Here's how the part is built. I have some questions about the finished solid (model axes, mm). Round coordinates to 2 decimals unless told otherwise and drop trailing zeros. Order: outer loops, then holes, each group sorted by start corner. A loop starts at its lowest first (then second) coordinate and runs counter-clockwise, first axis right, second up.
```python
from build123d import *

# Parameters (mm, degrees)
VACIADO2_T            = -2
CROQUIS2_R            = 3
CORTAR_EXTRUIR1_DEPTH = 26.980762114


with BuildPart() as part:
    # Croquis1 → Revolución1 (revolve)
    with BuildSketch(Plane.XY):
        with BuildLine():
            Line((0, 0), (0, 15))
            ThreePointArc((0, 15), (-10.606601718, 10.606601718), (-15, 0))
            Line((-15, 0), (0, 0))
        make_face()
    revolve(axis=Axis((0, 0, 0), (0, 1, 0)))

    # Vaciado2
    vaciado2_openings = [part.faces().sort_by_distance(p)[0] for p in [
        (0, 0, 0),
    ]]
    offset(amount=VACIADO2_T, openings=vaciado2_openings, kind=Kind.INTERSECTION)

    # Croquis2 → Cortar-Extruir1 (cut, through all)
    with BuildSketch(Plane.XY):
        with Locations(Location((0, 8.456456299, 0), (0, 0, 111.940512479))):
            Circle(CROQUIS2_R)
    extrude(amount=CORTAR_EXTRUIR1_DEPTH, mode=Mode.SUBTRACT)


solid = part.part
```
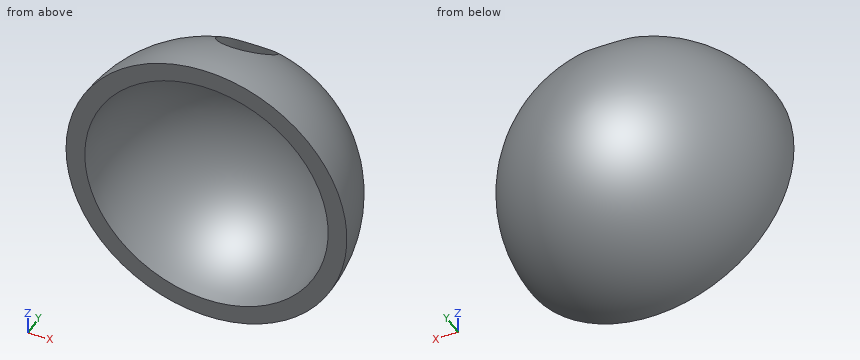
1. I need wall thicknesses on probe 1 along X at (y, z) = (4, 4); probe 2 along X at (y, z) = (11, -0.5); probe 3 along Z at (x, y) = (-10, 3.25). Which ranges of each line are inside material? Lowest first, please.
Evaluation:
probe 1: x = -13.89 to -11.7, 11.7 to 13.89
probe 2: x = -10.19 to -6.91, 6.91 to 10.19
probe 3: z = -10.7 to -7.64, 7.64 to 10.7
2. I'm going to push flat-ended pins straight in: P1, Ø2, axis at y = 9, z = -8.5, coming from the +X side; P2, Ø12, axis at x = -11.5, z = -11, coming from the +Y side; P3, Ø1, axis at y = 4, z = -9.5, coming from the +X side. Where does each tip first touch, or does it pass through?
Evaluation:
P1: stops at x = 9.77
P2: stops at y = 11.26
P3: stops at x = 11.35
3. If we section it at D-D, the plane y = 7.75: Write out the boundary of the cut face in (x, z), and give its area (3 significant figures).
Evaluation:
outline: (-2.92, 10.02) - (-2.92, 12.51) arc R12.84 ccw (long way) to (2.92, 12.51) - (2.92, 10.02) arc R10.44 cw (long way) to start
area: 162 mm2
4. If we section it at B-B, the plane z = 11.5: Write out the boundary of the cut face in (x, y).
Evaluation:
outline: (-9.63, 0) - (-6.06, 0) arc R6.06 cw to (-1.52, 5.87) arc R3 cw to (-2.91, 9.18) arc R9.63 ccw to start; (1.52, 5.87) arc R6.06 cw to (6.06, 0) - (9.63, 0) arc R9.63 ccw to (2.91, 9.18) arc R3 cw to start
5. If we section it at A-A, the plane x = 0: Write out the boundary of the cut face in (y, z).
Evaluation:
outline: (0, -15) arc R15 ccw to (11.46, 9.68) - (11.46, 6.14) arc R13 cw to (0, -13) - close; (0, 13) arc R13 cw to (5.46, 11.8) - (5.46, 13.97) arc R15 ccw to (0, 15) - close
6. If we section it at C-C, the plane y = 4.5: Write out the boundary of the cut face in (x, z), and give its area (3 significant figures).
Evaluation:
outline: circle Ø28.62 at (0, 0); hole circle Ø24.39 at (0, 0)
area: 176 mm2
